from build123d import *

# Parameters (mm, degrees)
IZIM1_R                     = 62.2
IZIM1_R_2                   = 59.2
Y_KSEKLIK_EKSTR_ZYON1_DEPTH = 100
DAIRESEL_KAPLAMA1_COUNT     = 4


with BuildPart() as part:
    # Çizim1 → Yükseklik-Ekstrüzyon1 (new, symmetric)
    with BuildSketch(Plane(origin=(0, 0, 0), x_dir=(1, 0, 0), z_dir=(0, 1, 0))):
        with Locations(Location((0, 0, 0), (0, 0, 270))):
            Circle(IZIM1_R)
        with Locations(Location((0, 0, 0), (0, 0, 270))):
            Circle(IZIM1_R_2, mode=Mode.SUBTRACT)
    extrude(amount=Y_KSEKLIK_EKSTR_ZYON1_DEPTH, both=True)

    # Çizim10 → M5 Boşluklu Delik1 (revolve, cut)
    with BuildSketch(Plane(origin=(62.2, -90, 0), x_dir=(0, 0, -1), z_dir=(0, 1, 0))):
        Polygon((0, 0), (0, 10.29228064), (2.65, 8.7), (2.65, 0), align=None)
    m5_bo_luklu_delik1 = revolve(axis=Axis((68.55, -90, 0), (-1, 0, 0)), mode=Mode.SUBTRACT)

    # Dairesel Kaplama1: M5 Boşluklu Delik1 ×4 about axis
    dairesel_kaplama1_axis = Axis((0, -100, 0), (0, 1, 0))
    for i in range(1, DAIRESEL_KAPLAMA1_COUNT):
        add(m5_bo_luklu_delik1.rotate(dairesel_kaplama1_axis, i * 360 / DAIRESEL_KAPLAMA1_COUNT), mode=Mode.SUBTRACT)


solid = part.part
Source: CAD feature listing. Evaluate the final solid. Frame: model axes, mm. Round coordinates to 2 decimals unless told otherwise and drop trailing zeros. Loops run counter-clockwise (first coordinate to the right, second up) from the corner with the lowest first, then second, coordinate; pieces in that order, holes last. Notation, with made-up numbers: M 54,33 L 93,33 A20 ccw 93,54 Z; hole C 57,70 d7. An arc over 180 degrees is marked long. Answer as CSV lines item,"result".
Q1. Cut plane A-A (x = 0). Return the cut outline in (y, z).
Verdict:
outline,"M -100,-62.2 L -92.65,-62.2 L -92.65,-59.2 L -100,-59.2 Z; M -100,59.2 L -92.65,59.2 L -92.65,62.2 L -100,62.2 Z; M -87.35,-62.2 L 100,-62.2 L 100,-59.2 L -87.35,-59.2 Z; M -87.35,59.2 L 100,59.2 L 100,62.2 L -87.35,62.2 Z"
Q2. Contact query for flat-ended pins moving along their axis: pin 1 (4 mm diameter, centred on x = -3, y = -61.5, fed in from +Z); pin 2 (8 mm diameter, centred on y = 13, z = 36, fed in from +X); pin 3 (5 mm diameter, centred on x = 0, y = -90, fed in from -Z); pin 4 (2 mm diameter, centred on x = -31, y = -48, fed in from -Z). Output: stop coordinate, or through.
Verdict:
pin 1,"stops at z = 62.19"
pin 2,"stops at x = 53.34"
pin 3,"passes through"
pin 4,"stops at z = -54.49"
Q3. Cut plane D-D (z = 15). Return the cut outline in (x, y), plus the area to 3 significant figures.
Verdict:
outline,"M -60.36,-100 L -57.27,-100 L -57.27,100 L -60.36,100 Z; M 57.27,-100 L 60.36,-100 L 60.36,100 L 57.27,100 Z"
area,"1,240 mm^2"
Q4. Cut plane B-B (z = 0). Return the cut outline in (x, y), plus the area to 3 significant figures.
Verdict:
outline,"M -62.2,-100 L -59.2,-100 L -59.2,-92.65 L -62.2,-92.65 Z; M -62.2,-87.35 L -59.2,-87.35 L -59.2,100 L -62.2,100 Z; M 59.2,-100 L 62.2,-100 L 62.2,-92.65 L 59.2,-92.65 Z; M 59.2,-87.35 L 62.2,-87.35 L 62.2,100 L 59.2,100 Z"
area,"1,170 mm^2"
Q5. Cut plane C-C (x = 50). Return the cut outline in (y, z).
Verdict:
outline,"M -100,-37 L 100,-37 L 100,-31.7 L -100,-31.7 Z; M -100,31.7 L 100,31.7 L 100,37 L -100,37 Z"
Q6. Line query: line 1 along Z through (x, y) = (0.5, -69); line 2 along Y through (x, z) = (61, 0); line 3 along Z through (x, y) = (21, -77). Output: solid intervals per line, ascending.
Verdict:
line 1,"z = -62.2 to -59.2, 59.2 to 62.2"
line 2,"y = -100 to -92.65, -87.35 to 100"
line 3,"z = -58.55 to -55.35, 55.35 to 58.55"
Q7. Pull-direction query (Z, two-part tool) for faces 1 (the face through (-23, -100, 55)), 2 (the face through (-55.182, 1.4, 28.702)), 3 (the face through (60.69, -87.41, 0.57)); classes: +Z half, -Z half, draft (parallel to the pull), parting line (faces both ways), or undercut.
Verdict:
face 1,"draft"
face 2,"parting line"
face 3,"undercut"
